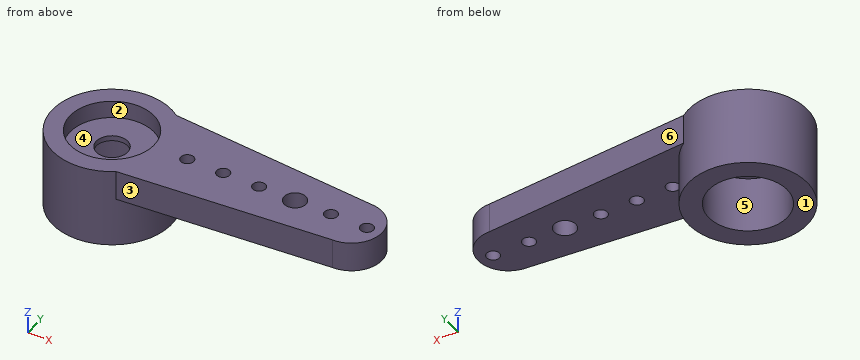
from build123d import *

# Parameters (mm, degrees)
SKICA1_R                 = 3.4
P_IDAT_VYSUNUT_M1_DEPTH  = 4.5
SKICA2_R                 = 2.25
ODEBRAT_VYSUNUT_M1_DEPTH = 3.2
SKICA3_R                 = 2.4
ODEBRAT_VYSUNUT_M2_DEPTH = 1
SKICA4_R                 = 0.9
ODEBRAT_VYSUNUT_M3_DEPTH = 0.3
P_IDAT_VYSUNUT_M2_DEPTH  = 1.7
SKICA6_R                 = 0.375
ODEBRAT_VYSUNUT_M4_DEPTH = 1.7
LINPOLE1_COUNT           = 6
LINPOLE1_PITCH           = 2.1
SKICA7_R                 = 0.625
ODEBRAT_VYSUNUT_M5_DEPTH = 1.7


with BuildPart() as part:
    # Skica1 → Přidat vysunutím1 (new body)
    with BuildSketch(Plane.XY):
        Circle(SKICA1_R)
    extrude(amount=P_IDAT_VYSUNUT_M1_DEPTH)

    # Skica2 → Odebrat vysunutím1 (cut)
    with BuildSketch(Plane(origin=(0, 0, 0), x_dir=(-1, 0, 0), z_dir=(0, 0, -1))):
        Circle(SKICA2_R)
    extrude(amount=-ODEBRAT_VYSUNUT_M1_DEPTH, mode=Mode.SUBTRACT)

    # Skica3 → Odebrat vysunutím2 (cut)
    with BuildSketch(Plane.XY.offset(4.5)):
        Circle(SKICA3_R)
    extrude(amount=-ODEBRAT_VYSUNUT_M2_DEPTH, mode=Mode.SUBTRACT)

    # Skica4 → Odebrat vysunutím3 (cut)
    with BuildSketch(Plane.XY.offset(3.5)):
        Circle(SKICA4_R)
    extrude(amount=-ODEBRAT_VYSUNUT_M3_DEPTH, mode=Mode.SUBTRACT)

    # Skica5 → Přidat vysunutím2 (add)
    with BuildSketch(Plane.XY.offset(4.5)):
        with BuildLine():
            Line((1.999374902, -2.75), (14, -1.75))
            ThreePointArc((14, -1.75), (15.75, 0), (14, 1.75))
            Line((14, 1.75), (1.999374902, 2.75))
            ThreePointArc((1.999374902, 2.75), (3.4, 0), (1.999374902, -2.75))
        make_face()
    extrude(amount=-P_IDAT_VYSUNUT_M2_DEPTH)

    # Skica6 → Odebrat vysunutím4 (cut)
    with BuildSketch(Plane.XY.offset(4.5)):
        with Locations((4.4, 0)):
            Circle(SKICA6_R)
    odebrat_vysunut_m4 = extrude(amount=-ODEBRAT_VYSUNUT_M4_DEPTH, mode=Mode.SUBTRACT)

    # LinPole1: Odebrat vysunutím4 ×6
    with Locations(*[(i * LINPOLE1_PITCH, 0, 0) for i in range(1, LINPOLE1_COUNT)]):
        add(odebrat_vysunut_m4, mode=Mode.SUBTRACT)

    # Skica7 → Odebrat vysunutím5 (cut)
    with BuildSketch(Plane.XY.offset(4.5)):
        with Locations((10.7, 0)):
            Circle(SKICA7_R)
    extrude(amount=-ODEBRAT_VYSUNUT_M5_DEPTH, mode=Mode.SUBTRACT)


solid = part.part
Build history of the part. All positions in model axes, mm. Face numbers are marked on the shaded views. A direction names the side the tool comes from. Give positions to 0.01 mm unless a question says otherwise; leave off trailing zeros. Loops run counter-clockwise (first coordinate to the right, second up) from the corner with the lowest first, then second, coordinate; pieces in that order, holes last. Notation, with made-up numbers: (52, 2) - (71, 2) arc R33 ccw to (71, 37) - close; hole circle Ø6 at (82.5, 56.25). An arc over 180 degrees is marked (long way). Write item = value, one per line. Start each with the question number.
1) Band-saw the part on C-C on y = -1.5. Give the cut face in (x, z).
2) Probe probe 1 along Z at (x, y) = (5, 1); probe 2 along X at (y, z) = (-1, 0.8); probe 3 along X at (y, z) = (-0.75, 3.7). List the from-to ranges inside material, lowest first. Write a range as from..to.
3) Band-saw the part on A-A on x = 12.8. Give the cut face in (y, z) (3 decimals), plus the area to 3 significant figures.
4) Tool access for the marked faces 4, 5 and 6: list every direction of +Z, -Z, +X, -X, +Y, -Y with a clear straight run to the whole face (end or side of a thin tool).
5) Drop flat-ended pins along their axis: pin 1 Ø1.5 at (y, z) = (2, 1) entering from +X; pin 2 Ø3.5 at (x, y) = (0, 0) entering from +Z; pin 3 Ø2 at (x, y) = (5.5, 0) entering from -Z. Give the stop position or say it passes through.
6) Pull direction Y, two halves, no side cores. Call the marked faces 1, 2 and 3: +Y half, -Y half, draft (parallel to the pull), parting line (faces both ways), or undercut.
7) Band-saw the part on B-B on z = 3.7. Give the cut face in (x, y) (3 decimals).
8) Band-saw the part on D-D on z = 1.5. Give the cut face in (x, y).
Final values:
q1.outline = (-3.05, 0) - (-1.68, 0) - (-1.68, 3.2) - (1.68, 3.2) - (1.68, 0) - (3.05, 0) - (3.05, 2.8) - (14.9, 2.8) - (14.9, 4.5) - (1.87, 4.5) - (1.87, 3.5) - (-1.87, 3.5) - (-1.87, 4.5) - (-3.05, 4.5) - close
q2.probe_1 = 2.8..4.5
q2.probe_2 = -3.25..-2.02, 2.02..3.25
q2.probe_3 = -3.32..-2.28, 2.28..15.58
q3.outline = (-1.85, 2.8) - (-0.375, 2.8) - (-0.375, 4.5) - (-1.85, 4.5) - close; (0.375, 2.8) - (1.85, 2.8) - (1.85, 4.5) - (0.375, 4.5) - close
q3.area = 5.01 mm²
q4.face_4 = +Z
q4.face_5 = -Z
q4.face_6 = +Z, -Z, +X, +Y
q5.pin_1 = 3.16
q5.pin_2 = 3.5
q5.pin_3 = 2.8
q6.face_1 = draft
q6.face_2 = undercut
q6.face_3 = -Y half
q7.outline = (1.999, -2.75) - (14, -1.75) arc R1.75 ccw to (14, 1.75) - (1.999, 2.75) arc R3.4 ccw (long way) to start; hole circle Ø4.8 at (0, 0); hole circle Ø0.75 at (4.4, 0); hole circle Ø0.75 at (6.5, 0); hole circle Ø0.75 at (8.6, 0); hole circle Ø1.25 at (10.7, 0); hole circle Ø0.75 at (12.8, 0); hole circle Ø0.75 at (14.9, 0)
q8.outline = circle Ø6.8 at (0, 0); hole circle Ø4.5 at (0, 0)
